Autodesk Inventor part; units mm, degrees
ref_plane "YZ Plane" through (0, 0, 0) normal (1, 0, 0) x (0, 1, 0)
ref_plane "XZ Plane" through (0, 0, 0) normal (0, 1, 0) x (-1, 0, 0)
ref_plane "XY Plane" through (0, 0, 0) normal (0, 0, 1) x (1, 0, 0)
sketch "Sketch1" plane through (0, 0, 0) normal (0, 0, 1) x (1, 0, 0)
  circle A0 centre (0, 0) radius 29
  circle A1 centre (0, 0) radius 27
  circle A2 centre (0, 0) radius 37
  dimension "d0" = 58
  dimension "d1" = 2
  dimension "d2" = 8
extrude "Extrusion1" add sketch "Sketch1" along normal blind 1.6 contours A0 | A2
sketch "Sketch2" plane through (0, 0, 1.6) normal (0, 0, 1) x (1, 0, 0)
  circle A0 centre (-32.9998, -0.1189) radius 1.25
  circle A1 centre (-16.3969, -28.6381) radius 1.25
  circle A2 centre (-16.6029, 28.5192) radius 1.25
  circle A3 centre (16.3969, 28.6381) radius 1.25
  circle A4 centre (16.6029, -28.5192) radius 1.25
  circle A5 centre (32.9998, 0.1189) radius 1.25
  circle A6 centre (-32.9998, -0.1189) radius 1.65
  circle A7 centre (-16.3969, -28.6381) radius 1.65
  circle A8 centre (16.6029, -28.5192) radius 1.65
  circle A9 centre (32.9998, 0.1189) radius 1.65
  circle A10 centre (16.3969, 28.6381) radius 1.65
  circle A11 centre (-16.6029, 28.5192) radius 1.65
  point P0 (0, 0)
  dimension "d5" = 3.3
  dimension "d8" = 360
extrude "Extrusion2" cut sketch "Sketch2" against normal through all contours A0 | A1 | A2 | A3 | A4 | A5 | A6 | A7 | A8 | A9 | A10 | A11
properties part number "stator_mount_ret"
Input: part model. Units: mm. Frame: model coordinates. Give positions to 0.01 mm unless a question says otherwise; leave off trailing zeros. Loops run counter-clockwise (first coordinate to the right, second up) from the corner with the lowest first, then second, coordinate; pieces in that order, holes last.
1) Contact query for a flat-ended pin moving along its axis: pin 1 (4.5 mm diameter, centred on x = -16.4, y = -28.64, fed in from -Z). Output: stop coordinate, or through.
A:
pin 1: stops at z = 0
2) Section query A-A on x = 0. Return the cut outline in (y, z), and give its area (3 significant figures).
A:
outline: (-37, 0) - (-27, 0) - (-27, 1.6) - (-37, 1.6) - close; (27, 0) - (37, 0) - (37, 1.6) - (27, 1.6) - close
area: 32.0 mm2
3) Mould query, pull axis X, two halves, no side actions, for faces 1 (the flat face through (-11, 25, 1.6)), 2 (the cylindrical face through (-8.02, 36.12, 0.79)), 3 (the cylindrical face through (-5.85, 26.36, 0.79)). Classes: released by +X, released by -X, zero draft, split by the parting line, or undercut.
A:
face 1: zero draft
face 2: split by the parting line
face 3: undercut
4) Section query C-C on z = 1.3. Return the cut outline in (x, y), and give its area (3 significant figures).
A:
outline: circle Ø74 at (0, 0); hole circle Ø3.3 at (-33, -0.12); hole circle Ø54 at (0, 0); hole circle Ø3.3 at (-16.6, 28.52); hole circle Ø3.3 at (-16.4, -28.64); hole circle Ø3.3 at (16.4, 28.64); hole circle Ø3.3 at (16.6, -28.52); hole circle Ø3.3 at (33, 0.12)
area: 1,960 mm2
5) Section query D-D on x = -28. Return the cut outline in (y, z), and give its area (3 significant figures).
A:
outline: (-24.19, 0) - (24.19, 0) - (24.19, 1.6) - (-24.19, 1.6) - close
area: 77.4 mm2
6) Line query: L1, parallel to X at y = 28, z = 1.4; L2, parallel to Y at x = 17, z = 0.35; L3, parallel to Y at x = 14, z = 0.25. Output: solid intervals per line, ascending.
A:
L1: x = -24.19 to -18.17, -15.04 to 14.88, 17.92 to 24.19
L2: y = -32.86 to -30.12, -26.92 to -20.98, 20.98 to 27.1, 30.17 to 32.86
L3: y = -34.25 to -23.09, 23.09 to 34.25
7) Section query B-B on y = 14.5. Return the cut outline in (x, z).
A:
outline: (-34.04, 0) - (-22.78, 0) - (-22.78, 1.6) - (-34.04, 1.6) - close; (22.78, 0) - (34.04, 0) - (34.04, 1.6) - (22.78, 1.6) - close
